Read the model definition and answer for the solid it produces. Units are mm, in the model's axes. Face numbers are marked on the shaded views. Give positions to 0.01 mm unless a question says otherwise; leave off trailing zeros. Loops run counter-clockwise (first coordinate to the right, second up) from the corner with the lowest first, then second, coordinate; pieces in that order, holes last. Notation, with made-up numbers: (5, -2.75) -> (47, -2.75) arc R27 ccw to (47, 20.25) -> close; hole circle Ø8 at (28, 35.5). An arc over 180 degrees is marked (long way). One line per item, written item: value. Start each with the question number.
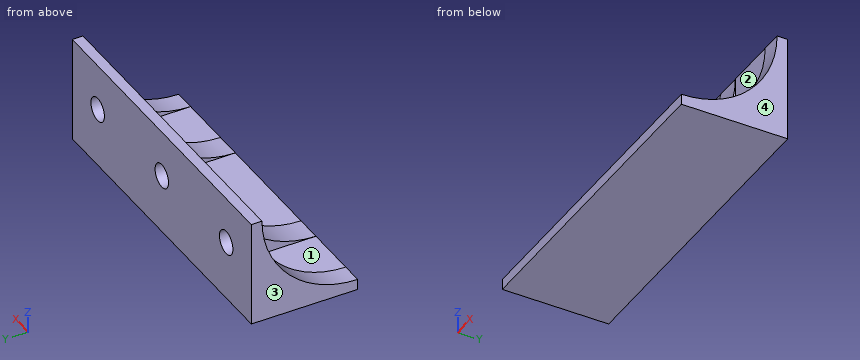
from build123d import *

# Parameters (mm, degrees)
SKETCH_1_W          = 60
SKETCH_1_H          = 20
EXTRUDE_1_DEPTH     = 2
SKETCH_2_W          = 60
SKETCH_2_H          = 2
EXTRUDE_2_DEPTH     = 18
FILLET_1_R          = 18
SKETCH_4_W          = 10
SKETCH_4_H          = 18
SKETCH_4_W_2        = 22
CUT_EXTRUDE_1_DEPTH = 18
HOLE_WIZARD_M4_1_D  = 4.5


with BuildPart() as part:
    # 스케치1 → 보스-돌출1 (new body)
    with BuildSketch(Plane.XY):
        Rectangle(SKETCH_1_W, SKETCH_1_H)
    extrude(amount=EXTRUDE_1_DEPTH)

    # 스케치2 → 보스-돌출2 (add)
    with BuildSketch(Plane.XY.offset(2)):
        with Locations((0, 9)):
            Rectangle(SKETCH_2_W, SKETCH_2_H)
    extrude(amount=EXTRUDE_2_DEPTH)

    # 필렛1
    fillet_1_edges = [part.edges().sort_by_distance(p)[0] for p in [
        (0, 8, 2),
    ]]
    fillet(fillet_1_edges, radius=FILLET_1_R - 0.0001)  # a hair under: the kernel refuses the full size

    # 스케치4 → 컷-돌출1 (cut)
    with BuildSketch(Plane.XY.offset(20)):
        with Locations((-21, -1)):
            Rectangle(SKETCH_4_W, SKETCH_4_H)
        with Locations((0, -1)):
            Rectangle(SKETCH_4_W_2, SKETCH_4_H)
        with Locations((21, -1)):
            Rectangle(SKETCH_4_W, SKETCH_4_H)
    extrude(amount=-CUT_EXTRUDE_1_DEPTH, mode=Mode.SUBTRACT)

    # M4 여유 구멍1 (through all)
    with Locations(Plane(origin=(0, 8, 0), x_dir=(-1, 0, 0), z_dir=(0, -1, 0))):
        with Locations((-21.498688558, -11.191274161), (21.579331698, -11.191274161), (0, -11.191274161)):
            Hole(HOLE_WIZARD_M4_1_D / 2)


solid = part.part
Item 1: Section B-B, the plane z = 12.75 is taken. Determine the outline of the cut face in (x, y), plus the area to 3 significant figures.
Item 2: Consider L1, parallel to X at y = -3, z = 2.75; L2, parallel to Z at x = 0, y = 8.9; L3, parallel to Z at x = 24.5, y = 5.25. Determine where each line is inside the solid, lowest interval first. Write a range as [from, to].
Item 3: Section A-A, the plane x = 0 is taken. Determine the outline of the cut face in (y, z).
Item 4: Flat-ended cylindrical pins translate along their axes: pin 1 (1 mm diameter, centred on x = 4, z = 4.5, fed in from -Y); pin 2 (4 mm diameter, centred on x = -3, y = 5, fed in from +Z). Find the tip coordinate at first contact, or state that the pin passes through.
Item 5: Section C-C, the plane y = 9.25 is taken. Determine the outline of the cut face in (x, z), plus the area to 3 significant figures.
Item 6: Determine the mould class of the marked faces 1, 2, 3 and 4 for opening direction X: pulls with the +X half, pulls with the -X half, needs draft (parallel to the pull), parting line crosses it, or undercut.
Item 7: Section D-D, the plane y = -2 is taken. Determine the outline of the cut face in (x, z), plus the area to 3 significant figures.
Computed values:
1. outline: (-30, 6.48) -> (-26, 6.48) -> (-26, 8) -> (-23.2, 8) -> (-23.2, 10) -> (-30, 10) -> close; (-19.96, 8) -> (-16, 8) -> (-16, 6.48) -> (-11, 6.48) -> (-11, 8) -> (-1.62, 8) -> (-1.62, 10) -> (-19.96, 10) -> close; (1.62, 8) -> (11, 8) -> (11, 6.48) -> (16, 6.48) -> (16, 8) -> (19.88, 8) -> (19.88, 10) -> (1.62, 10) -> close; (23.12, 8) -> (26, 8) -> (26, 6.48) -> (30, 6.48) -> (30, 10) -> (23.12, 10) -> close
1. area: 128 mm²
2. L1: [-30, -26], [-16, -11], [11, 16], [26, 30]
2. L2: [0, 8.94], [13.44, 20]
2. L3: [0, 2]
3. outline: (-10, 0) -> (10, 0) -> (10, 8.94) -> (8, 8.94) -> (8, 2) -> (-10, 2) -> close; (8, 13.44) -> (10, 13.44) -> (10, 20) -> (8, 20) -> close
4. pin 1: y = 8
4. pin 2: z = 2
5. outline: (-30, 0) -> (30, 0) -> (30, 20) -> (-30, 20) -> close; hole circle Ø4.5 at (-21.58, 11.19); hole circle Ø4.5 at (0, 11.19); hole circle Ø4.5 at (21.5, 11.19)
5. area: 1,150 mm²
6. face 1: undercut
6. face 2: undercut
6. face 3: pulls with the -X half
6. face 4: pulls with the +X half
7. outline: (-30, 0) -> (30, 0) -> (30, 3.88) -> (26, 3.88) -> (26, 2) -> (16, 2) -> (16, 3.88) -> (11, 3.88) -> (11, 2) -> (-11, 2) -> (-11, 3.88) -> (-16, 3.88) -> (-16, 2) -> (-26, 2) -> (-26, 3.88) -> (-30, 3.88) -> close
7. area: 154 mm²
